Geometry: see drawing. Coordinates: mm, zero at the bounding-box minimum. A direction names the side the tool comes from. Round coordinates to 2 decimals unless told otherwise and drop trailing zeros. Loops run counter-clockwise (first coordinate to the right, second up) from the corner with the lowest first, then second, coordinate; pieces in that order, holes last. Notation, with made-up numbers: M 28,-2 L 68,-2 A22 ccw 68,22 Z; hole C 26.25,-9.5 d9. An arc over 180 degrees is marked long. Answer as a JSON object with one key per item and string values.
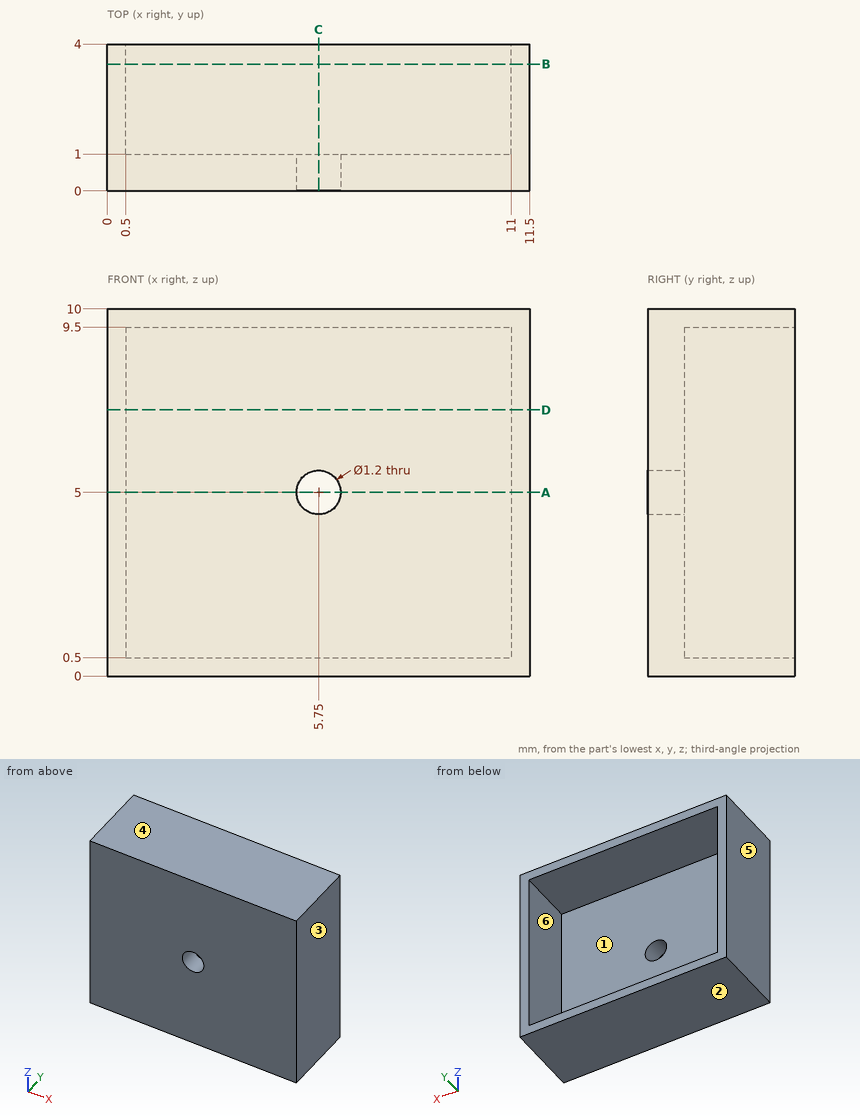
1) Section query C-C (x = 5.75). Return the cut outline in (y, z).
Results:
{"outline": "M 0,0 L 4,0 L 4,0.5 L 1,0.5 L 1,4.4 L 0,4.4 Z; M 0,5.6 L 1,5.6 L 1,9.5 L 4,9.5 L 4,10 L 0,10 Z"}
2) Reachability of the marked faces 1 and 2 from +Z, -Z, +X, -X, +Y, -Y: full face, straight path, thin tool, end or side. Return the list, or none.
Results:
{"face 1": "+Y", "face 2": "-Z, +X, -X, +Y, -Y"}
3) Pull-direction query (X, two-part tool) for the marked faces 3, 4, 5 and 6; classes: +X half, -X half, draft (parallel to the pull), parting line (faces both ways), or undercut.
Results:
{"face 3": "+X half", "face 4": "draft", "face 5": "-X half", "face 6": "undercut"}
4) Section query B-B (y = 3.45). Return the cut outline in (x, z).
Results:
{"outline": "M 0,0 L 11.5,0 L 11.5,10 L 0,10 Z; hole M 0.5,0.5 L 11,0.5 L 11,9.5 L 0.5,9.5 Z"}
5) Section query D-D (z = 7.25). Return the cut outline in (x, y), and give its area (3 significant figures).
Results:
{"outline": "M 0,0 L 11.5,0 L 11.5,4 L 11,4 L 11,1 L 0.5,1 L 0.5,4 L 0,4 Z", "area": "14.5 mm2"}
6) Pin query (flat end, axial travel): P1, Ø1, axis at y = 2, z = 7.5, coming from the -X side. Return the tip coordinate at first contact, or that it passes through.
Results:
{"P1": "x = 0"}
7) Section query A-A (z = 5). Return the cut outline in (x, y), and give its area (3 significant figures).
Results:
{"outline": "M 0,0 L 5.15,0 L 5.15,1 L 0.5,1 L 0.5,4 L 0,4 Z; M 6.35,0 L 11.5,0 L 11.5,4 L 11,4 L 11,1 L 6.35,1 Z", "area": "13.3 mm2"}
8) Ray query, line 1 (X direction, y = 0.45, z = 5); line 2 (Z direction, x = 5.75, y = 0.85); line 3 (Z direction, x = 3.75, y = 2.5). Return the intervals inside material, ascending.
Results:
{"line 1": "0 to 5.15, 6.35 to 11.5", "line 2": "0 to 4.4, 5.6 to 10", "line 3": "0 to 0.5, 9.5 to 10"}
